Work out the finished part from the listing and answer in its coordinate system (mm). A direction names the side the tool comes from. Coordinates: 2 decimals unless noted, no trailing zeros. Loops run counter-clockwise (first coordinate to the right, second up) from the corner with the lowest first, then second, coordinate; pieces in that order, holes last. Notation, with made-up numbers: (79, 11) -> (104, 11) arc R34 ccw to (104, 50) -> close; hole circle Ø5 at (55, 74). An arc over 180 degrees is marked (long way). Use a Markdown table: item, result. Add a question column.
```python
from build123d import *

# Parameters (mm, degrees)
SKETCH_1_W          = 30
SKETCH_1_H          = 30
SKETCH_1_W_2        = 28
SKETCH_1_H_2        = 28
EXTRUDE_1_DEPTH     = 40
SKETCH_2_R          = 1.5
CUT_EXTRUDE_1_DEPTH = 53.201532545
SKETCH_3_R          = 1.5
CUT_EXTRUDE_2_DEPTH = 53.201532545


with BuildPart() as part:
    # 草图1 → 凸台-拉伸1 (new body)
    with BuildSketch(Plane.XY):
        Rectangle(SKETCH_1_W, SKETCH_1_H)
        Rectangle(SKETCH_1_W_2, SKETCH_1_H_2, mode=Mode.SUBTRACT)
    extrude(amount=EXTRUDE_1_DEPTH)

    # 草图2 → 切除-拉伸1 (cut, through all)
    with BuildSketch(Plane.ZY.offset(15)):
        with Locations((32, -7)):
            Circle(SKETCH_2_R)
        with Locations((8, -7)):
            Circle(SKETCH_2_R)
        with Locations((32, 7)):
            Circle(SKETCH_2_R)
        with Locations((8, 7)):
            Circle(SKETCH_2_R)
    extrude(amount=-CUT_EXTRUDE_1_DEPTH, mode=Mode.SUBTRACT)

    # 草图3 → 切除-拉伸2 (cut, through all)
    with BuildSketch(Plane(origin=(0, 15, 0), x_dir=(1, 0, 0), z_dir=(0, 1, 0))):
        with Locations(Location((7, -32, 0), (0, 0, 270))):
            Circle(SKETCH_3_R)
        with Locations(Location((-7, -32, 0), (0, 0, 270))):
            Circle(SKETCH_3_R)
        with Locations(Location((7, -8, 0), (0, 0, 270))):
            Circle(SKETCH_3_R)
        with Locations(Location((-7, -8, 0), (0, 0, 270))):
            Circle(SKETCH_3_R)
    extrude(amount=-CUT_EXTRUDE_2_DEPTH, mode=Mode.SUBTRACT)


solid = part.part
```
Item 1: For a pull along Z with two mould halves and no side action, classify faces 1 (the face through (-7.9, 14.5, 6.8)), 2 (the face through (-1.2, -14.4, 0)), 3 (the face through (0, -15, 20)), 4 (the face through (14.5, -7.9, 6.8)) as +Z half, -Z half, draft (parallel to the pull), parting line (faces both ways), or undercut.
Item 2: Section A-A (x = -7) is taken. Determine the outline of the cut face in (y, z).
Item 3: Given pin 1 (1.5 mm diameter, centred on x = -2.5, y = 12, fed in from +Z), flat-ended and moving along its own axis, determine where the tip first touches the part or whether it passes through.
Item 4: Section C-C (z = 34) is taken. Determine the outline of the cut face in (x, y), then the cut area to 3 significant figures.
Item 5: Section B-B (x = -10.5) is taken. Determine the outline of the cut face in (y, z).
Item 6: For faces 5 (the face through (14, 0, 20)), 6 (the face through (-14.5, 6.1, 6.8)), determine the directions among +Z, -Z, +X, -X, +Y, -Y from which every point of the face is accessible in a straight line to the end or side of a thin tool.
Item 7: Find the intervals of material crossed by probe 1 along X at (y, z) = (-14.15, 32); probe 2 along Y at (x, z) = (-0.75, 34.5), in increasing order.
Output:
| question | item | result |
|---|---|---|
| 1 | face 1 | undercut |
| 1 | face 2 | -Z half |
| 1 | face 3 | draft |
| 1 | face 4 | undercut |
| 2 | outline | (-15, 0) -> (-14, 0) -> (-14, 6.5) -> (-15, 6.5) -> close; (-15, 9.5) -> (-14, 9.5) -> (-14, 30.5) -> (-15, 30.5) -> close; (-15, 33.5) -> (-14, 33.5) -> (-14, 40) -> (-15, 40) -> close; (14, 0) -> (15, 0) -> (15, 6.5) -> (14, 6.5) -> close; (14, 9.5) -> (15, 9.5) -> (15, 30.5) -> (14, 30.5) -> close; (14, 33.5) -> (15, 33.5) -> (15, 40) -> (14, 40) -> close |
| 3 | pin 1 | passes through |
| 4 | outline | (-15, -15) -> (15, -15) -> (15, 15) -> (-15, 15) -> close; hole (-14, -14) -> (14, -14) -> (14, 14) -> (-14, 14) -> close |
| 4 | area | 116 mm2 |
| 5 | outline | (-15, 0) -> (-14, 0) -> (-14, 40) -> (-15, 40) -> close; (14, 0) -> (15, 0) -> (15, 40) -> (14, 40) -> close |
| 6 | face 5 | +Z, -Z |
| 6 | face 6 | +X, -X |
| 7 | probe 1 | x = -15 to -8.5, -5.5 to 5.5, 8.5 to 15 |
| 7 | probe 2 | y = -15 to -14, 14 to 15 |
